Could you check a few things on this model? Use its own coordinates, in mm. A direction names the side the tool comes from. Coordinates: 2 decimals unless noted, no trailing zeros. Loops run counter-clockwise (first coordinate to the right, second up) from the corner with the lowest first, then second, coordinate; pieces in that order, holes last.
from build123d import *

# Parameters (mm, degrees)
F0_R     = 2.5
F1_DEPTH = 10
F2_R     = 6.5
F2_R_2   = 2.5
F3_DEPTH = 25
F4_R     = 2.5
F5_ANGLE = 45
F6_W     = 30
F6_H     = 10
F6_R     = 2.5
F7_DEPTH = 60
F8_SIZE2 = 5
F8_SIZE  = 5


with BuildPart() as f1:
    # F0 (on Top) → F1 (new body)
    with BuildSketch(Plane.XY):
        Circle(F0_R)
    extrude(amount=F1_DEPTH)

    # F2 (on face) → F3 (join)
    with BuildSketch(Plane.XY.offset(10)):
        Circle(F2_R)
        Circle(F2_R_2, mode=Mode.SUBTRACT)
        Circle(F2_R_2)
    extrude(amount=F3_DEPTH)

    # F4 (on face) → F5 (revolve)
    with BuildSketch(Plane.XY.offset(35)):
        Circle(F4_R)
    revolve(axis=Axis((1.7774057342, -7.2282995097, 35), (1, 0, 0)), revolution_arc=F5_ANGLE)

    # F6 (on face) → F7 (join)
    with BuildSketch(Plane(origin=(0, -21.1141497549, 21.1141497549), x_dir=(1, 0, 0), z_dir=(0, -0.7071067812, 0.7071067812))):
        with Locations((0, 26.8658572515)):
            Rectangle(F6_W, F6_H)
        with Locations((0, 26.8658572515)):
            Circle(F6_R, mode=Mode.SUBTRACT)
        with Locations((0, 26.8658572515)):
            Circle(F6_R)
    extrude(amount=F7_DEPTH)

    # F8
    f8_edges = [f1.edges().sort_by_distance(p)[0] for p in [
        (0, -41.007993, 86.07312),
        (-15, -44.543527, 82.537586),
        (15, -44.543527, 82.537586),
    ]]
    chamfer(f8_edges, length=F8_SIZE, length2=F8_SIZE2)


solid = f1.part
1) We'd pull the mould along Z, two halves only. Please class faces 3 (the flat face through (3, 0, 35)), 4 (the flat face through (15, -21, 59)), 5 (the flat face through (-0.21, -17.755, 62.82)): released by +Z, released by -Z, zero draft, split by the parting line, or undercut.
2) Imagine slicing it at D-D on x = 1.5. List the corners of the cut face in (y, z) for me.
3) Imagine slicing it at B-B on z = 11. List the corners of the cut face in (x, y) for me.
4) For faces 1 (the cylindrical face through (-5.158, -3.955, 22.325)), 2 (the flat face through (-15, -21, 59)), which set-ups out of +Z, -Z, +X, -X, +Y, -Y let a thin tool reach every point of the face, with its end or its side?
5) If I drill on L1, parallel to Z at x = 1, y = -3; L2, parallel to Y at x = -4, z = 31.5; L3, parallel to Z at x = -7, y = -36.5, over which ranges is the centre line in solid material (lowest first)?
6) Imagine slicing it at C-C on y = -16.5. List the corners of the cut face in (x, z) for me, plus the area to 3 significant figures.
7) Will these pins go through, and if not, where does the flat tip stop? pin 1 (10 mm diameter, centred on x = 9, y = -18.5, fed in from +Z); pin 2 (1.5 mm diameter, centred on x = -4.5, y = -41, fed in from -Z); pin 3 (14.5 mm diameter, centred on x = 2, y = 3, fed in from +Z).
8) Imagine slicing it at A-A on x = -9. List the corners of the cut face in (y, z) for me.
Solved:
1. face 3: undercut
1. face 4: zero draft
1. face 5: released by +Z
2. outline: (-48.08, 79) - (-5.65, 36.58) - (-3.53, 38.7) arc R5.23 cw to (-2, 35) - (-6.32, 35) - (-6.32, 10) - (-2, 10) - (-2, 0) - (2, 0) - (2, 10) - (6.32, 10) - (6.32, 35) - (2, 35) arc R9.23 ccw to (-0.7, 41.53) - (1.42, 43.65) - (-37.47, 82.54) - (-44.54, 82.54) - close
3. outline: circle Ø13 at (0, 0)
4. face 1: -Z
4. face 2: +Z, -Z, -X, +Y, -Y
5. L1: z = 10 to 35, 37.55 to 48.07
5. L2: y = -5.12 to 5.12
5. L3: z = 67.42 to 81.57
6. outline: (-15, 47.42) - (15, 47.42) - (15, 61.57) - (-15, 61.57) - close
6. area: 424 mm2
7. pin 1: stops at z = 68.57
7. pin 2: stops at z = 71.17
7. pin 3: stops at z = 49.32
8. outline: (-48.08, 79) - (-5.65, 36.58) - (1.42, 43.65) - (-37.47, 82.54) - (-44.54, 82.54) - close
